from build123d import *

# Parameters (mm, degrees)
F0_W      = 25
F0_H      = 40
F1_DEPTH  = 40
F2_W      = 22
F2_H      = 37
F3_DEPTH  = 40.001
F5_DEPTH  = 1
F6_R      = 1.35
F7_DEPTH  = 40.001
F8_W      = 3
F8_H      = 22
F9_DEPTH  = 25.001
F10_R     = 1.2
F11_R     = 0.75
F12_DEPTH = 25.001


with BuildPart() as f1:
    # F0 (on Top) → F1 (new body)
    with BuildSketch(Plane.XY):
        Rectangle(F0_W, F0_H)
    extrude(amount=F1_DEPTH)

    # F2 (on face) → F3 (cut, through all)
    with BuildSketch(Plane.XY.offset(40)):
        Rectangle(F2_W, F2_H)
    extrude(amount=-F3_DEPTH, mode=Mode.SUBTRACT)

    # F4 (on face) → F5 (join)
    with BuildSketch(Plane(origin=(0, 0, 0), x_dir=(1, 0, 0), z_dir=(0, 0, -1))):
        with BuildLine():
            Line((-11, 18.5), (-11, 11))
            ThreePointArc((-11, 11), (-5.696699, 13.196699), (-3.5, 18.5))
            Line((-3.5, 18.5), (-11, 18.5))
        make_face()
        with BuildLine():
            Line((11, 18.5), (3.5, 18.5))
            ThreePointArc((3.5, 18.5), (5.696699, 13.196699), (11, 11))
            Line((11, 11), (11, 18.5))
        make_face()
        with BuildLine():
            Line((11, -18.5), (11, -11))
            ThreePointArc((11, -11), (5.696699, -13.196699), (3.5, -18.5))
            Line((3.5, -18.5), (11, -18.5))
        make_face()
        with BuildLine():
            Line((-11, -18.5), (-3.5, -18.5))
            ThreePointArc((-3.5, -18.5), (-5.696699, -13.196699), (-11, -11))
            Line((-11, -11), (-11, -18.5))
        make_face()
    extrude(amount=-F5_DEPTH)

    # F6 (on face) → F7 (cut, through all)
    with BuildSketch(Plane(origin=(0, 0, 0), x_dir=(1, 0, 0), z_dir=(0, 0, -1))):
        with Locations((7.5, 15)):
            Circle(F6_R)
        with Locations((-7.5, 15)):
            Circle(F6_R)
        with Locations((7.5, -15)):
            Circle(F6_R)
        with Locations((-7.5, -15)):
            Circle(F6_R)
    extrude(amount=-F7_DEPTH, mode=Mode.SUBTRACT)

    # F8 (on face) → F9 (cut, through all)
    with BuildSketch(Plane.YZ.offset(12.5)):
        with Locations((-6.5, 11)):
            Rectangle(F8_W, F8_H)
        with Locations((6.5, 11)):
            Rectangle(F8_W, F8_H)
        with BuildLine():
            Line((-1.5, 40), (-1.5, 23.5))
            ThreePointArc((-1.5, 23.5), (0, 22), (1.5, 23.5))
            Line((1.5, 23.5), (1.5, 40))
            Line((1.5, 40), (-1.5, 40))
        make_face()
    extrude(amount=-F9_DEPTH, mode=Mode.SUBTRACT)

    # F10
    f10_edges = [f1.edges().sort_by_distance(p)[0] for p in [
        (11.75, -5, 22),
        (-11.75, -5, 22),
        (11.75, -8, 22),
        (-11.75, -8, 22),
        (11.75, 5, 22),
        (-11.75, 5, 22),
        (11.75, 8, 22),
        (-11.75, 8, 22),
    ]]
    fillet(f10_edges, radius=F10_R)

    # F11 (on face) → F12 (cut, through all)
    with BuildSketch(Plane.YZ.offset(12.5)):
        with Locations((-3, 10)):
            Circle(F11_R)
        with Locations((0, 10)):
            Circle(F11_R)
        with Locations((3, 10)):
            Circle(F11_R)
    extrude(amount=-F12_DEPTH, mode=Mode.SUBTRACT)


solid = f1.part
Design review of the part built by this model. Coordinates are the model's own, in mm. A direction names the side the tool comes from. Coordinates: 2 decimals unless noted, no trailing zeros. Write each loop counter-clockwise with the first axis right and the second up, starting at its lowest first coordinate (ties: lowest second). Pieces come first, ordered by that corner, then holes. Notation, with made-up numbers: (67, 68) - (98, 68) arc R10 ccw to (98, 76) - close; hole circle Ø9 at (30, 45.5). An arc over 180 degrees is marked (long way). Use one line per item in the form item = value.
Q1. Consider section B-B (z = 12). Write out the cut boundary in (x, y), plus the area to 3 significant figures.
Taken from the geometry:
outline = (-12.5, -20) - (12.5, -20) - (12.5, -8) - (11, -8) - (11, -18.5) - (-11, -18.5) - (-11, -8) - (-12.5, -8) - close; (-12.5, -5) - (-11, -5) - (-11, 5) - (-12.5, 5) - close; (-12.5, 8) - (-11, 8) - (-11, 18.5) - (11, 18.5) - (11, 8) - (12.5, 8) - (12.5, 20) - (-12.5, 20) - close; (11, -5) - (12.5, -5) - (12.5, 5) - (11, 5) - close
area = 168 mm^2
Q2. For probe 1 along Y at (x, z) = (7.25, 7.5); probe 2 along Y at (x, z) = (-7.5, 0.45); probe 3 along X at (y, z) = (3, 29), list the stretches that pass through material, from the lowest coordinate up.
Taken from the geometry:
probe_1 = -20 to -18.5, 18.5 to 20
probe_2 = -20 to -16.35, -13.65 to -11.87, 11.87 to 13.65, 16.35 to 20
probe_3 = -12.5 to -11, 11 to 12.5
Q3. Consider section C-C (x = 1). Write out the cut boundary in (y, z).
Taken from the geometry:
outline = (-20, 0) - (-18.5, 0) - (-18.5, 40) - (-20, 40) - close; (18.5, 0) - (20, 0) - (20, 40) - (18.5, 40) - close
Q4. Consider section D-D (z = 31.5). Write out the cut boundary in (x, y).
Taken from the geometry:
outline = (-12.5, -20) - (12.5, -20) - (12.5, -1.5) - (11, -1.5) - (11, -18.5) - (-11, -18.5) - (-11, -1.5) - (-12.5, -1.5) - close; (-12.5, 1.5) - (-11, 1.5) - (-11, 18.5) - (11, 18.5) - (11, 1.5) - (12.5, 1.5) - (12.5, 20) - (-12.5, 20) - close
Q5. Machinability: for faces 1 (the cylindrical face through (11.74, -5.342, 21.639)), 2 (the flat face through (0, 18.5, 20)), 3 (the cylindrical face through (-5.755, -13.139, 0.493)), which of the approach directions +Z, -Z, +X, -X, +Y, -Y give a long, thin tool a straight path to every point of the face, cutting with its end or side? Answer none if there is none.
Taken from the geometry:
face_1 = -Z, +X, -X
face_2 = +Z
face_3 = +Z, -Z
Q6. Consider section A-A (y = 9). Write out the cut boundary in (x, z), plus the area to 3 significant figures.
Taken from the geometry:
outline = (-12.5, 0) - (-11, 0) - (-11, 40) - (-12.5, 40) - close; (11, 0) - (12.5, 0) - (12.5, 40) - (11, 40) - close
area = 120 mm^2
Q7. Insertion check: pin 1 Ø0.5 at (x, y) = (12, 6.5) entering from -Z; pin 2 Ø2.5 at (y, z) = (3, 10) entering from +X; pin 3 Ø2.5 at (x, y) = (-6.5, -15.5) entering from +Z. Each pin has a flat end and moves straight along its axis. Give the tip position at first contact, or say it passes through.
Taken from the geometry:
pin_1 = 22
pin_2 = 12.5
pin_3 = 1
